Input: part model. Units: mm. Frame: model coordinates. A direction names the side the tool comes from. Give positions to 0.01 mm unless a question says otherwise; leave off trailing zeros. Order: outer loops, then holes, each group sorted by start corner. A loop starts at its lowest first (then second) coordinate and runs counter-clockwise, first axis right, second up. Notation, with made-up numbers: (8, 12.25) - (38, 12.25) arc R24 cw to (38, 44.25) - close; hole circle Ø11 at (46.25, 69). An arc over 180 degrees is marked (long way). Use a Markdown table: item, result.
from build123d import *

# Parameters (mm, degrees)
SKETCH1_W                = 26
SKETCH1_H                = 15
BOSS_EXTRUDE1_DEPTH      = 7
BOSS_EXTRUDE1_DEPTH_BACK = 7
SKETCH3_R                = 3.04
CUT_EXTRUDE1_DEPTH       = 7
CUT_EXTRUDE1_DEPTH_BACK  = 7
SKETCH4_R                = 4
CUT_EXTRUDE2_DEPTH       = 5
CHAMFER1_SIZE            = 3
FILLET1_R                = 2
ESQUISSE1_R              = 2.75
ENL_V_MAT_EXTRU_1_DEPTH  = 10
ESQUISSE2_R              = 2.75
ENL_V_MAT_EXTRU_2_DEPTH  = 10


with BuildPart() as part:
    # Sketch1 → Boss-Extrude1 (new body, two sides)
    with BuildSketch(Plane.XY) as boss_extrude1_sk:
        Rectangle(SKETCH1_W, SKETCH1_H)
    extrude(amount=BOSS_EXTRUDE1_DEPTH)
    extrude(boss_extrude1_sk.sketch, amount=-BOSS_EXTRUDE1_DEPTH_BACK)

    # Sketch3 → Cut-Extrude1 (cut, two sides)
    with BuildSketch(Plane.XY) as cut_extrude1_sk:
        with Locations((0, -1.5)):
            Circle(SKETCH3_R)
    extrude(amount=CUT_EXTRUDE1_DEPTH, mode=Mode.SUBTRACT)
    extrude(cut_extrude1_sk.sketch, amount=-CUT_EXTRUDE1_DEPTH_BACK, mode=Mode.SUBTRACT)

    # Sketch4 → Cut-Extrude2 (cut)
    with BuildSketch(Plane(origin=(0, 7.5, 0), x_dir=(1, 0, 0), z_dir=(0, 1, 0))):
        with Locations((-6.5, 0)):
            Circle(SKETCH4_R)
        with Locations((6.5, 0)):
            Circle(SKETCH4_R)
    extrude(amount=-CUT_EXTRUDE2_DEPTH, mode=Mode.SUBTRACT)

    # Chamfer1
    chamfer1_edges = [part.edges().sort_by_distance(p)[0] for p in [
        (13, 0, -7),
        (-13, 0, 7),
        (13, 0, 7),
        (-13, 0, -7),
    ]]
    chamfer(chamfer1_edges, length=CHAMFER1_SIZE)

    # Fillet1
    fillet1_edges = [part.edges().sort_by_distance(p)[0] for p in [
        (13, 0, 4),
        (13, 0, -4),
        (-10, 0, -7),
        (10, 0, -7),
        (-10, 0, 7),
        (10, 0, 7),
        (-13, 0, 4),
        (-13, 0, -4),
    ]]
    fillet(fillet1_edges, radius=FILLET1_R)

    # Esquisse1 → Enl_v. mat.-Extru.1 (cut)
    with BuildSketch(Plane(origin=(0, 2.5, 0), x_dir=(1, 0, 0), z_dir=(0, 1, 0))):
        with Locations((6.5, 0)):
            Circle(ESQUISSE1_R)
    extrude(amount=-ENL_V_MAT_EXTRU_1_DEPTH, mode=Mode.SUBTRACT)

    # Esquisse2 → Enl_v. mat.-Extru.2 (cut)
    with BuildSketch(Plane(origin=(0, 2.5, 0), x_dir=(1, 0, 0), z_dir=(0, 1, 0))):
        with Locations((-6.5, 0)):
            Circle(ESQUISSE2_R)
    extrude(amount=-ENL_V_MAT_EXTRU_2_DEPTH, mode=Mode.SUBTRACT)


solid = part.part
1. Section query D-D (y = -3). Return loops of the section in (x, z).
Response:
| item | result |
|---|---|
| outline | (-13, -3.17) arc R2 ccw to (-12.41, -4.59) - (-10.59, -6.41) arc R2 ccw to (-9.17, -7) - (-2.64, -7) - (-2.64, 7) - (-9.17, 7) arc R2 ccw to (-10.59, 6.41) - (-12.41, 4.59) arc R2 ccw to (-13, 3.17) - close; (2.64, -7) - (9.17, -7) arc R2 ccw to (10.59, -6.41) - (12.41, -4.59) arc R2 ccw to (13, -3.17) - (13, 3.17) arc R2 ccw to (12.41, 4.59) - (10.59, 6.41) arc R2 ccw to (9.17, 7) - (2.64, 7) - close; hole circle Ø5.5 at (-6.5, 0); hole circle Ø5.5 at (6.5, 0) |
2. Pin query (flat end, axial travel): pin 1 (4 mm diameter, centred on y = -1.5, z = -3.5, fed in from -X); pin 2 (5 mm diameter, centred on x = -6.5, z = 0, fed in from -Y); pin 3 (6.5 mm diameter, centred on x = 6.5, z = 0, fed in from +Y). Return the tip coordinate at first contact, or that it passes through.
Response:
| item | result |
|---|---|
| pin 1 | stops at x = -13 |
| pin 2 | passes through |
| pin 3 | stops at y = 2.5 |
3. Section query B-B (z = -1.5). Return loops of the section in (x, y), then the cut area to 3 significant figures.
Response:
| item | result |
|---|---|
| outline | (-13, -7.5) - (-8.8, -7.5) - (-8.8, 2.5) - (-10.21, 2.5) - (-10.21, 7.5) - (-13, 7.5) - close; (-4.2, -7.5) - (4.2, -7.5) - (4.2, 2.5) - (2.79, 2.5) - (2.79, 7.5) - (-2.79, 7.5) - (-2.79, 2.5) - (-4.2, 2.5) - close; (8.8, -7.5) - (13, -7.5) - (13, 7.5) - (10.21, 7.5) - (10.21, 2.5) - (8.8, 2.5) - close; hole circle Ø6.08 at (0, -1.5) |
| area | 195 mm^2 |
4. Section query A-A (y = 5). Return loops of the section in (x, z).
Response:
| item | result |
|---|---|
| outline | (-13, -3.17) arc R2 ccw to (-12.41, -4.59) - (-10.59, -6.41) arc R2 ccw to (-9.17, -7) - (9.17, -7) arc R2 ccw to (10.59, -6.41) - (12.41, -4.59) arc R2 ccw to (13, -3.17) - (13, 3.17) arc R2 ccw to (12.41, 4.59) - (10.59, 6.41) arc R2 ccw to (9.17, 7) - (-9.17, 7) arc R2 ccw to (-10.59, 6.41) - (-12.41, 4.59) arc R2 ccw to (-13, 3.17) - close; hole circle Ø8 at (-6.5, 0); hole circle Ø8 at (6.5, 0) |
5. Material intervals for line 1 along Y through (x, z) = (0, 0.75); line 2 along X through (y, z) = (-2, 2.25); line 3 along X through (y, z) = (6.75, -1.5), sorted ascending.
Response:
| item | result |
|---|---|
| line 1 | y = -7.5 to -4.54, 1.54 to 7.5 |
| line 2 | x = -13 to -8.08, -4.92 to -3, 3 to 4.92, 8.08 to 13 |
| line 3 | x = -13 to -10.21, -2.79 to 2.79, 10.21 to 13 |
6. Mould query, pull axis X, two halves, no side actions, for faces 3 (the face through (-9.947, 0.105, -6.844)), 4 (the face through (9.93, 0.11, 6.85)), 5 (the face through (5.633, 5.035, 3.905)), 6 (the face through (9.04, -2.43, 1.05)). Classes: pulls with the +X half, pulls with the -X half, needs draft (parallel to the pull), parting line crosses it, or undercut.
Response:
| item | result |
|---|---|
| face 3 | pulls with the -X half |
| face 4 | pulls with the +X half |
| face 5 | undercut |
| face 6 | undercut |
7. Set-up query: faces 1 (the face through (-7.367, 5.035, 3.905)), 2 (the face through (13, 0, 0)). Return all of +Z, -Z, +X, -X, +Y, -Y with unobstructed straight access to the full face (end or side cutting, diameter ignored); none if empty.
Response:
| item | result |
|---|---|
| face 1 | +Y |
| face 2 | +Z, -Z, +X, +Y, -Y |
8. Section query C-C (x = -6.5). Return loops of the section in (y, z), then the cut area to 3 significant figures.
Response:
| item | result |
|---|---|
| outline | (-7.5, -7) - (7.5, -7) - (7.5, -4) - (2.5, -4) - (2.5, -2.75) - (-7.5, -2.75) - close; (-7.5, 2.75) - (2.5, 2.75) - (2.5, 4) - (7.5, 4) - (7.5, 7) - (-7.5, 7) - close |
| area | 115 mm^2 |
